from build123d import *

# Parameters (mm, degrees)
EXTRUDE_1_DEPTH     = 4
SKETCH_2_R          = 1.6
CUT_EXTRUDE_1_DEPTH = 5
CUT_EXTRUDE_2_DEPTH = 5
FILLET_1_R          = 2


with BuildPart() as part:
    # 草图1 → 凸台-拉伸1 (new body)
    with BuildSketch(Plane.XY):
        Polygon((-25, 0), (25, 0), (25, 20), (35, 20), (35, 30), (-35, 30), (-35, 20), (-25, 20), align=None)
    extrude(amount=EXTRUDE_1_DEPTH)

    # 草图2 → 切除-拉伸1 (cut, through all)
    with BuildSketch(Plane.XY.offset(4)):
        with Locations((19, 10)):
            Circle(SKETCH_2_R)
        with Locations((19, 25)):
            Circle(SKETCH_2_R)
        with Locations((-19, 10)):
            Circle(SKETCH_2_R)
        with Locations((-19, 25)):
            Circle(SKETCH_2_R)
    extrude(amount=-CUT_EXTRUDE_1_DEPTH, mode=Mode.SUBTRACT)

    # 草图3 → 切除-拉伸2 (cut, through all)
    with BuildSketch(Plane.XY.offset(4)):
        with BuildLine():
            Line((-7.2, 17.3), (7.2, 17.3))
            ThreePointArc((7.2, 17.3), (14.5, 10), (7.2, 2.7))
            Line((7.2, 2.7), (-7.2, 2.7))
            ThreePointArc((-7.2, 2.7), (-14.5, 10), (-7.2, 17.3))
        make_face()
    extrude(amount=-CUT_EXTRUDE_2_DEPTH, mode=Mode.SUBTRACT)

    # 圆角1
    fillet_1_edges = [part.edges().sort_by_distance(p)[0] for p in [
        (-25, 20, 2),
        (-35, 20, 2),
        (-35, 30, 2),
        (35, 30, 2),
        (35, 20, 2),
        (25, 20, 2),
        (25, 0, 2),
        (-25, 0, 2),
    ]]
    fillet(fillet_1_edges, radius=FILLET_1_R)


solid = part.part
The model under review builds one solid part; all positions refer to its coordinate system, in mm. A direction names the side the tool comes from. Give positions to 0.01 mm unless a question says otherwise; leave off trailing zeros. Loops run counter-clockwise (first coordinate to the right, second up) from the corner with the lowest first, then second, coordinate; pieces in that order, holes last. Notation, with made-up numbers: (50, 81.5) -> (92, 81.5) arc R35 ccw to (92, 119.5) -> close; hole circle Ø7 at (83, 64.5). An arc over 180 degrees is marked (long way). Write each question's results on one line, items separated by ' | '.
1) For line 1 along Y through (x, z) = (19, 2.3); line 2 along Y through (x, z) = (-20, 1.8); line 3 along X through (y, z) = (17.75, 2.2), list the stretches that pass through material, from the lowest coordinate up. Write a range as from..to.
Conclusion:
line 1: y = 0..8.4, 11.6..23.4, 26.6..30 | line 2: y = 0..8.75, 11.25..23.75, 26.25..30 | line 3: x = -25..25
2) Draft analysis for pull direction X (two halves, no side actions). For faces 1 (the face through (0, 17.3, 2)), 2 (the face through (35, 25, 2)), 3 (the face through (-34.43, 29.4, 2.03)), state which applies: pulls with the +X half, pulls with the -X half, needs draft (parallel to the pull), parting line crosses it, or undercut.
Conclusion:
face 1: undercut | face 2: pulls with the +X half | face 3: pulls with the -X half
3) Take a section at C-C, the plane y = 10. Give the boundary of the cut face in (x, z), plus the area to 3 significant figures.
Conclusion:
outline: (-25, 0) -> (-20.6, 0) -> (-20.6, 4) -> (-25, 4) -> close; (-17.4, 0) -> (-14.5, 0) -> (-14.5, 4) -> (-17.4, 4) -> close; (14.5, 0) -> (17.4, 0) -> (17.4, 4) -> (14.5, 4) -> close; (20.6, 0) -> (25, 0) -> (25, 4) -> (20.6, 4) -> close | area: 58.4 mm^2
4) Take a section at D-D, the plane x = -10. Give the boundary of the cut face in (y, z).
Conclusion:
outline: (0, 0) -> (3.26, 0) -> (3.26, 4) -> (0, 4) -> close; (16.74, 0) -> (30, 0) -> (30, 4) -> (16.74, 4) -> close
5) Take a section at A-A, the plane y = 25. Give the boundary of the cut face in (x, z).
Conclusion:
outline: (-35, 0) -> (-20.6, 0) -> (-20.6, 4) -> (-35, 4) -> close; (-17.4, 0) -> (17.4, 0) -> (17.4, 4) -> (-17.4, 4) -> close; (20.6, 0) -> (35, 0) -> (35, 4) -> (20.6, 4) -> close
6) Insertion check: pin 1 Ø1.2 at (x, z) = (30, 2) entering from -Y; pin 2 Ø3 at (x, y) = (19, 25) entering from +Z; pin 3 Ø1.2 at (y, z) = (10, 1.5) entering from -X; pin 4 Ø2 at (y, z) = (10, 2) entering from +X. Each pin has a flat end and moves straight along its axis. Give the tip position at first contact, or say it passes through.
Conclusion:
pin 1: stops at y = 20 | pin 2: passes through | pin 3: stops at x = -25 | pin 4: stops at x = 25
7) Take a section at B-B, the plane x = 19. Give the boundary of the cut face in (y, z), plus the area to 3 significant figures.
Conclusion:
outline: (0, 0) -> (8.4, 0) -> (8.4, 4) -> (0, 4) -> close; (11.6, 0) -> (23.4, 0) -> (23.4, 4) -> (11.6, 4) -> close; (26.6, 0) -> (30, 0) -> (30, 4) -> (26.6, 4) -> close | area: 94.4 mm^2
8) Tool access review of faces 4 (the face through (14.5, 10.16, 2.03)), 5 (the face through (-30, 20, 2)), 6 (the face through (25, 10, 2)), 7 (the face through (0, 30, 2)): name each direction out of +Z, -Z, +X, -X, +Y, -Y from which nothing blocks a thin tool from reaching the whole face with its end or side.
Conclusion:
face 4: +Z, -Z | face 5: +Z, -Z, -X, -Y | face 6: +Z, -Z, +X, -Y | face 7: +Z, -Z, +X, -X, +Y
